Design review of the part built by this model. Coordinates are the model's own, in mm. Round coordinates to 2 decimals unless told otherwise and drop trailing zeros. Write each loop counter-clockwise with the first axis right and the second up, starting at its lowest first coordinate (ties: lowest second). Pieces come first, ordered by that corner, then holes. Notation, with made-up numbers: M -21,-14 L 3,-14 A31 cw 3,18 Z; hole C 47,-21 d9. An arc over 180 degrees is marked long. Use CSV: the item, a comma, the result in double quotes.
from build123d import *

# Parameters (mm, degrees)
SKETCH1_R           = 31.75
SKETCH1_R_2         = 3.4925
BOSS_EXTRUDE1_DEPTH = 3.175
SKETCH2_R           = 2.667
CUT_EXTRUDE1_DEPTH  = 7.35


with BuildPart() as part:
    # Sketch1 → Boss-Extrude1 (new body, symmetric)
    with BuildSketch(Plane(origin=(0, 0, 0), x_dir=(1, 0, 0), z_dir=(0, 1, 0))):
        Circle(SKETCH1_R)
        Circle(SKETCH1_R_2, mode=Mode.SUBTRACT)
    extrude(amount=BOSS_EXTRUDE1_DEPTH, both=True)

    # Sketch2 → Cut-Extrude1 (cut, through all)
    with BuildSketch(Plane.XZ.offset(3.175)):
        with Locations((-17.78, 12.7)):
            Circle(SKETCH2_R)
        with Locations((-25.4, 0)):
            Circle(SKETCH2_R)
        with Locations((-17.78, -12.7)):
            Circle(SKETCH2_R)
        with Locations((17.78, -12.7)):
            Circle(SKETCH2_R)
        with Locations((25.4, 0)):
            Circle(SKETCH2_R)
        with Locations((17.78, 12.7)):
            Circle(SKETCH2_R)
    extrude(amount=-CUT_EXTRUDE1_DEPTH, mode=Mode.SUBTRACT)


solid = part.part
1) The part is to be moulded in two halves that separate along Z. For faces 1 (the face through (0, -3.175, 7)), 2 (the face through (15.66, -0.04, -14.32)), 3 (the face through (-6.883, 0.044, 30.995)), say which applies: released by +Z, released by -Z, zero draft, split by the parting line, or undercut.
Answers:
face 1,"zero draft"
face 2,"undercut"
face 3,"split by the parting line"
2) Add section D-D on x = 17.78. Write out the cut boundary in (y, z) (3 decimals).
Answers:
outline,"M -3.175,-26.305 L 3.175,-26.305 L 3.175,-15.367 L -3.175,-15.367 Z; M -3.175,-10.033 L 3.175,-10.033 L 3.175,10.033 L -3.175,10.033 Z; M -3.175,15.367 L 3.175,15.367 L 3.175,26.305 L -3.175,26.305 Z"
3) Add section B-B on z = 0. Give the number of separate pieces and of enclosed holes in the cut face, then the cut area to 3 significant figures.
Answers:
separate pieces,"4"
enclosed holes,"0"
area,"291 mm²"
4) Wall thickness on line 1 along Z through (x, y) = (-19, 1); line 2 along Z through (x, y) = (0, -0.25); line 3 along Z through (x, y) = (-17.78, -0.25): over which ranges is each line inside the solid? List them lowest first. Write a range as [from, to].
Answers:
line 1,"[-25.44, -15.07], [-10.33, 10.33], [15.07, 25.44]"
line 2,"[-31.75, -3.49], [3.49, 31.75]"
line 3,"[-26.3, -15.37], [-10.03, 10.03], [15.37, 26.3]"
5) For pin 1 Ø1 at (x, y) = (3, 1.5) entering from +Z; pin 2 Ø2 at (y, z) = (-1.5, 4.5) entering from -X, all flat-tipped, find the tip position at first contact; note any pin that passes through.
Answers:
pin 1,"z = 31.65"
pin 2,"x = -31.56"
